```python
from build123d import *

# Parameters (mm, degrees)
SKETCH1_W               = 33
SKETCH1_H               = 11
SKETCH1_R               = 1.75
BOSS_EXTRUDE1_DEPTH     = 10.5
CHAMFER1_SIZE           = 2
CUT_EXTRUDE1_DEPTH      = 66.570572836
CUT_EXTRUDE1_DEPTH_BACK = 66.570572836
SKETCH3_R               = 1.25
CUT_EXTRUDE2_DEPTH      = 20.5
CUT_EXTRUDE2_DEPTH_BACK = 20.5
SKETCH3_3_R             = 1.75
SKETCH3_3_R_2           = 1.25
CUT_EXTRUDE3_START      = 23.5
SKETCH3_6_R             = 1.25
CUT_EXTRUDE3_DEPTH      = 8
CUT_EXTRUDE4_START      = -15.5
SKETCH3_7_R             = 1.25
CUT_EXTRUDE4_DEPTH      = 8
CUT_EXTRUDE5_DEPTH      = 59.570470544
CUT_EXTRUDE5_DEPTH_BACK = 59.570470544
BOSS_EXTRUDE2_DEPTH     = 3


with BuildPart() as part:
    # Sketch1 → Boss-Extrude1 (new body)
    with BuildSketch(Plane(origin=(0, 0, 0), x_dir=(1, 0, 0), z_dir=(0, 1, 0))):
        with Locations((0, 11)):
            Rectangle(SKETCH1_W, SKETCH1_H)
        with Locations(Location((-10.5, 11, 0), (0, 0, 90))):
            Circle(SKETCH1_R, mode=Mode.SUBTRACT)
        with Locations(Location((10.5, 11, 0), (0, 0, 90))):
            Circle(SKETCH1_R, mode=Mode.SUBTRACT)
    extrude(amount=BOSS_EXTRUDE1_DEPTH)

    # Sketch2 → Loft1 section 0
    with BuildSketch(Plane(origin=(0, 41.5, 0), x_dir=(1, 0, 0), z_dir=(0, 1, 0))):
        with BuildLine():
            Line((-23.5, 45), (-16.5, 45))
            Line((-16.5, 45), (-16.5, 5))
            Line((-16.5, 5), (-23.5, 5))
            Line((-23.5, 5), (-23.5, 45))
        make_face()
    # Sketch1<3> → Loft1 section 1
    with BuildSketch(Plane(origin=(0, 0, 0), x_dir=(1, 0, 0), z_dir=(0, 1, 0))):
        with BuildLine():
            Line((-23.5, 45), (-16.5, 45))
            Line((-16.5, 45), (-16.5, 0))
            Line((-16.5, 0), (-23.5, 0))
            Line((-23.5, 0), (-23.5, 45))
        make_face()
    loft()

    # Sketch2<3> → Loft2 section 0
    with BuildSketch(Plane(origin=(0, 41.5, 0), x_dir=(1, 0, 0), z_dir=(0, 1, 0))):
        with BuildLine():
            Line((16.5, 45), (16.5, 5))
            Line((16.5, 5), (23.5, 5))
            Line((23.5, 5), (23.5, 45))
            Line((23.5, 45), (16.5, 45))
        make_face()
    # Sketch1<4> → Loft2 section 1
    with BuildSketch(Plane(origin=(0, 0, 0), x_dir=(1, 0, 0), z_dir=(0, 1, 0))):
        with BuildLine():
            Line((16.5, 45), (16.5, 0))
            Line((16.5, 0), (23.5, 0))
            Line((23.5, 0), (23.5, 45))
            Line((23.5, 45), (16.5, 45))
        make_face()
    loft()

    # Chamfer1
    chamfer1_edges = [part.edges().sort_by_distance(p)[0] for p in [
        (20, 41.5, -45),
        (-20, 41.5, -45),
    ]]
    chamfer(chamfer1_edges, length=CHAMFER1_SIZE)

    # Sketch3 → Cut-Extrude1 (cut, two sides: drawn at the far end of the back side and taken through both)
    with BuildSketch(Plane(origin=(0, 0, 0), x_dir=(0, 0, -1), z_dir=(1, 0, 0)).offset(-CUT_EXTRUDE1_DEPTH_BACK)):
        with Locations((7.25, 37.75)):
            Circle(SKETCH3_R)
        with Locations((42.25, 37.75)):
            Circle(SKETCH3_R)
        with Locations((42.25, 2.75)):
            Circle(SKETCH3_R)
    extrude(amount=CUT_EXTRUDE1_DEPTH + CUT_EXTRUDE1_DEPTH_BACK, mode=Mode.SUBTRACT)

    # Sketch3<3> → Cut-Extrude2 (cut, two sides: drawn at the far end of the back side and taken through both)
    # profile 1 of 3: a face of its own
    with BuildSketch(Plane(origin=(0, 0, 0), x_dir=(0, 0, -1), z_dir=(1, 0, 0)).offset(-CUT_EXTRUDE2_DEPTH_BACK)):
        with Locations(Location((7.25, 37.75, 0), (0, 0, 180))):
            Circle(SKETCH3_3_R)
        with Locations((7.25, 37.75)):
            Circle(SKETCH3_3_R_2, mode=Mode.SUBTRACT)
    # profile 2 of 3: a face of its own
    with BuildSketch(Plane(origin=(0, 0, 0), x_dir=(0, 0, -1), z_dir=(1, 0, 0)).offset(-CUT_EXTRUDE2_DEPTH_BACK)):
        with Locations(Location((42.25, 37.75, 0), (0, 0, 180))):
            Circle(SKETCH3_3_R)
        with Locations((42.25, 37.75)):
            Circle(SKETCH3_3_R_2, mode=Mode.SUBTRACT)
    # profile 3 of 3: a face of its own
    with BuildSketch(Plane(origin=(0, 0, 0), x_dir=(0, 0, -1), z_dir=(1, 0, 0)).offset(-CUT_EXTRUDE2_DEPTH_BACK)):
        with Locations(Location((42.25, 2.75, 0), (0, 0, 180))):
            Circle(SKETCH3_3_R)
        with Locations((42.25, 2.75)):
            Circle(SKETCH3_3_R_2, mode=Mode.SUBTRACT)
    extrude(amount=CUT_EXTRUDE2_DEPTH + CUT_EXTRUDE2_DEPTH_BACK, mode=Mode.SUBTRACT)

    # Sketch3<6> → Cut-Extrude3 (cut)
    with BuildSketch(Plane(origin=(0, 0, 0), x_dir=(0, 0, -1), z_dir=(1, 0, 0)).offset(CUT_EXTRUDE3_START)):
        with Locations((7.25, 2.75)):
            Circle(SKETCH3_6_R)
    extrude(amount=-CUT_EXTRUDE3_DEPTH, mode=Mode.SUBTRACT)

    # Sketch3<7> → Cut-Extrude4 (cut)
    with BuildSketch(Plane(origin=(0, 0, 0), x_dir=(0, 0, -1), z_dir=(1, 0, 0)).offset(CUT_EXTRUDE4_START)):
        with Locations((7.25, 2.75)):
            Circle(SKETCH3_7_R)
    extrude(amount=-CUT_EXTRUDE4_DEPTH, mode=Mode.SUBTRACT)

    # Sketch4 → Cut-Extrude5 (cut, two sides: drawn at the far end of the back side and taken through both)
    with BuildSketch(Plane.XY.offset(-11).offset(-CUT_EXTRUDE5_DEPTH_BACK)):
        with BuildLine():
            ThreePointArc((-6, 10.5), (0, 16.5), (6, 10.5))
            Line((6, 10.5), (8, 10.5))
            ThreePointArc((8, 10.5), (0, 18.5), (-8, 10.5))
            Line((-8, 10.5), (-6, 10.5))
        make_face()
        with BuildLine():
            Line((8, 10.5), (6, 10.5))
            ThreePointArc((6, 10.5), (0, 4.5), (-6, 10.5))
            Line((-6, 10.5), (-8, 10.5))
            ThreePointArc((-8, 10.5), (0, 2.5), (8, 10.5))
        make_face()
        with BuildLine():
            ThreePointArc((-6, 10.5), (0, 4.5), (6, 10.5))
            Line((6, 10.5), (-6, 10.5))
        make_face()
        with BuildLine():
            Line((-6, 10.5), (6, 10.5))
            ThreePointArc((6, 10.5), (0, 16.5), (-6, 10.5))
        make_face()
    extrude(amount=CUT_EXTRUDE5_DEPTH + CUT_EXTRUDE5_DEPTH_BACK, mode=Mode.SUBTRACT)

    # Sketch4<4> → Boss-Extrude2 (add, symmetric)
    with BuildSketch(Plane.XY.offset(-11)):
        with BuildLine():
            Line((8, 10.5), (6, 10.5))
            ThreePointArc((6, 10.5), (0, 4.5), (-6, 10.5))
            Line((-6, 10.5), (-8, 10.5))
            ThreePointArc((-8, 10.5), (0, 2.5), (8, 10.5))
        make_face()
    extrude(amount=BOSS_EXTRUDE2_DEPTH, both=True)


solid = part.part
```
Model file for the job. Use its own axes, mm. A direction names the side the tool comes from. Give positions to 0.01 mm unless a question says otherwise; leave off trailing zeros. Loops run counter-clockwise (first coordinate to the right, second up) from the corner with the lowest first, then second, coordinate; pieces in that order, holes last. Notation, with made-up numbers: (-7.75, -28.5) - (41.25, -28.5) arc R22 ccw to (41.25, -5.5) - close; hole circle Ø10 at (76, 21.25). An arc over 180 degrees is marked (long way). One line per item, written item: value. Start each with the question number.
1. Pull direction Y, two halves, no side cores. Call faces 6 (the cylindrical face through (-19.4, 2.8, -6)), 7 (the flat face through (0, 2, -5.5)), 8 (the flat face through (20, 40.5, -44)): pulls with the +Y half, pulls with the -Y half, needs draft (parallel to the pull), parting line crosses it, or undercut.
2. Slice it at D-D (x = 0). List the corners of the cut face in (y, z).
3. Which spindle directions (+Z, -Z, +X, -X, +Y, -Y) get a long thin tool onto all of the face, cutting with end or side? Do faces 1 (the flat face through (12.3, 10.5, -9.9)), 2 (the flat face through (19.951, 20.46, -2.465)), 3 (the flat face through (0, 2, -16.5)), 4 (the flat face through (0, 4, -8)), 5 (the cylindrical face through (-18.53, 39.3, -6.44)). Say none if no direction does.
4. Slice it at C-C (z = -11). Give the number of separate pieces and of enclosed holes in the cut face, plus the area to 3 significant figures.
5. Probe L1, parallel to Y at x = 19.6, z = -42.25; L2, parallel to Y at x = -21.25, z = -7.25; L3, parallel to X at y = 31, z = -5. List the from-to ranges inside material, lowest first. Write a range as from..to.
6. Pin check, flat tips, straight feed: pin 1 (2 mm diameter, centred on y = 2.75, z = -7.25, fed in from -X); pin 2 (11.5 mm diameter, centred on x = 10.5, z = -12.5, fed in from +Y). Stop position of each tip, or through.
7. Slice it at A-A (x = 19). List the corners of the cut face in (y, z), plus the area to 3 significant figures.
8. Slice it at B-B (x = -10.5). List the corners of the cut face in (y, z), plus the area to 4 significant figures.
Solution:
1. face 6: undercut
1. face 7: needs draft
1. face 8: pulls with the +Y half
2. outline: (0, -16.5) - (2.5, -16.5) - (2.5, -14) - (4.5, -14) - (4.5, -8) - (2.5, -8) - (2.5, -5.5) - (0, -5.5) - close
3. face 1: +Z, -Z, +Y
3. face 2: +Z, +X, -X, +Y
3. face 3: -Z, +Y, -Y
3. face 4: +Z, +Y
3. face 5: none
4. separate pieces: 3
4. enclosed holes: 0
4. area: 797 mm^2
5. L1: y = 0..1, 4.5..36, 39.5..41.5
5. L2: y = 0..1.5, 4..36.5, 39..41.5
5. L3: x = -23.5..-16.5, 16.5..23.5
6. pin 1: stops at x = -15.5
6. pin 2: stops at y = 10.5
7. outline: (0, -45) - (39.5, -45) - (41.5, -43) - (41.5, -5) - (0, 0) - close; hole circle Ø3.5 at (2.75, -42.25); hole circle Ø2.5 at (2.75, -7.25); hole circle Ø3.5 at (37.75, -42.25); hole circle Ø3.5 at (37.75, -7.25)
7. area: 1,730 mm^2
8. outline: (0, -16.5) - (10.5, -16.5) - (10.5, -12.75) - (0, -12.75) - close; (0, -9.25) - (10.5, -9.25) - (10.5, -5.5) - (0, -5.5) - close
8. area: 78.75 mm^2
